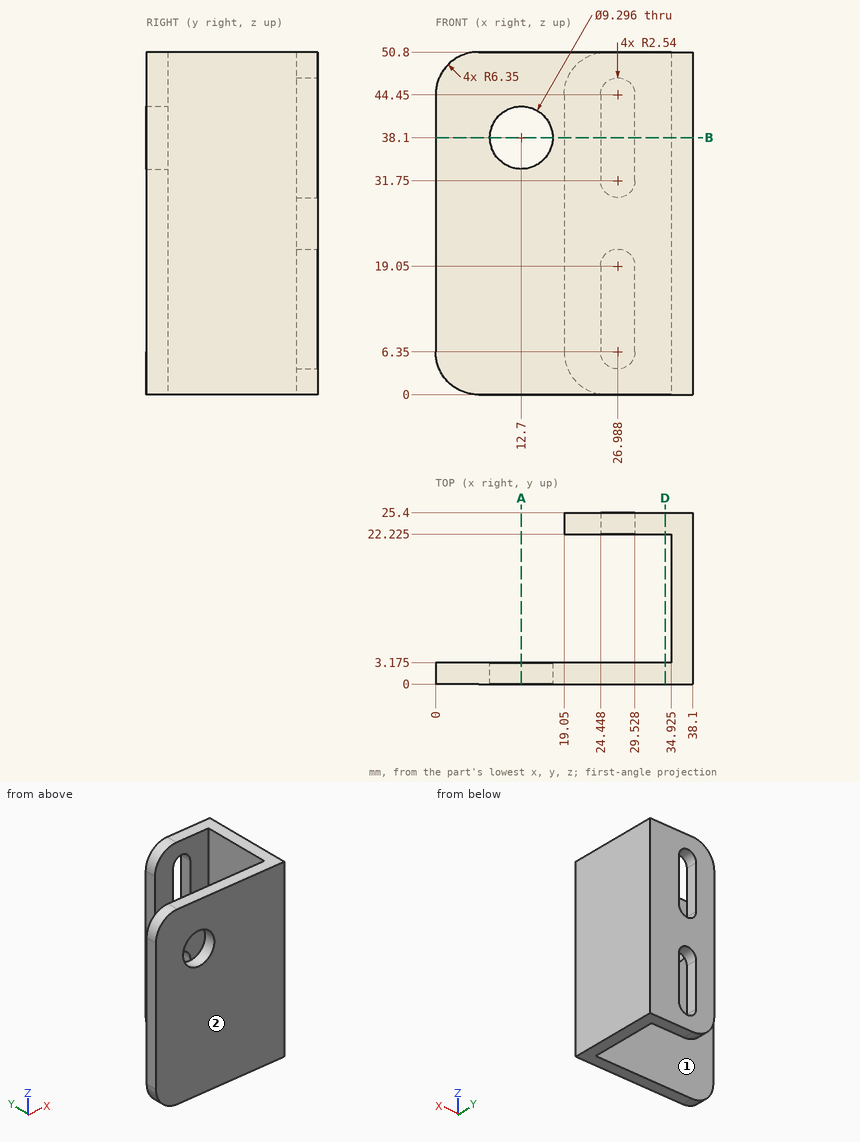
The drawing under review shows one solid part. Ordinate dimensions are in mm from its lowest x, y, z. A direction names the side the tool comes from. Coordinates: 2 decimals unless noted, no trailing zeros. Loops run counter-clockwise (first coordinate to the right, second up) from the corner with the lowest first, then second, coordinate; pieces in that order, holes last. Notation, with made-up numbers: (19.5, -21) - (70.5, -21) arc R24 ccw to (70.5, -2) - close; hole circle Ø5 at (47.25, 87.25). An arc over 180 degrees is marked (long way). Return JSON: item names as keys, results as strings.
Item 1: Take a section at D-D (x = 34). Give the boundary of the cut face in (y, z) (1 decimal).
Determined:
{"outline": "(0, 0) - (3.2, 0) - (3.2, 50.8) - (0, 50.8) - close; (22.2, 0) - (25.4, 0) - (25.4, 50.8) - (22.2, 50.8) - close"}
Item 2: Insertion check: pin 1 (3 mm diameter, centred on x = 17.5, z = 9.5, fed in from +Y) (1 decimal); pin 2 (1 mm diameter, centred on y = 24.5, z = 15, fed in from -X); pin 3 (5.5 mm diameter, centred on y = 8.5, z = 37, fed in from -X) (1 decimal). Each pin has a flat end and moves straight along its axis. Give the tip position at first contact, or say it passes through.
Determined:
{"pin 1": "stops at y = 3.2", "pin 2": "stops at x = 19.05", "pin 3": "stops at x = 34.9"}
Item 3: For line 1 (X direction, y = 23, z = 39); line 2 (Y direction, x = 29.5, z = 30) (1 decimal); line 3 (Z direction, x = 12.7, y = 1.8), list the stretches that pass through material, from the lowest coordinate up.
Determined:
{"line 1": "x = 19.05 to 24.45, 29.53 to 38.1", "line 2": "y = 0 to 3.2, 22.2 to 25.4", "line 3": "z = 0 to 33.45, 42.75 to 50.8"}
Item 4: For the marked faces 1 and 2, list the 3-axis set-ups (+Z, -Z, +X, -X, +Y, -Y) from which the entire face can be reached by the end or side of a thin tool; tool diameter is ignored.
Determined:
{"face 1": "+Z, -Z, -X", "face 2": "+Z, -Z, +X, -X, -Y"}
Item 5: Take a section at A-A (x = 12.7). Give the boundary of the cut face in (y, z) (1 decimal), then the cut area to 3 significant figures.
Determined:
{"outline": "(0, 0) - (3.2, 0) - (3.2, 33.5) - (0, 33.5) - close; (0, 42.7) - (3.2, 42.7) - (3.2, 50.8) - (0, 50.8) - close", "area": "132 mm2"}
Item 6: Take a section at B-B (z = 38.1). State how many separate pieces and enclosed holes the cut face has, then the cut area to 3 significant figures.
Determined:
{"separate pieces": "3", "enclosed holes": "0", "area": "196 mm2"}
